Drawing for the job (mm, zero at the part's lowest x, y, z). Give positions to 0.01 mm unless a question says otherwise; leave off trailing zeros. Loops run counter-clockwise (first coordinate to the right, second up) from the corner with the lowest first, then second, coordinate; pieces in that order, holes last.
1) Flat gauge pin, fed straight in: P1, Ø1.4, axis at y = 3, z = 56.857, coming from the +X side. Where does the tip first touch, or does it go through?
2) Band-saw the part on B-B on y = 7. List the corners of the cut face in (x, z), then the cut area to 3 significant figures.
3) Wall check: line 1 (Z direction, x = 0.7, y = 69); line 2 (Y direction, x = 0.95, z = 57); line 3 (Y direction, x = 4.1, z = 15). Give the ranges that are in metal, low to high.
4) Band-saw the part on C-C on x = 4.75. List the corners of the cut face in (y, z), then the cut area to 3 significant figures.
5) Band-saw the part on D-D on z = 32.5. List the corners of the cut face in (x, y).
6) Band-saw the part on A-A on y = 69. List the corners of the cut face in (x, z).
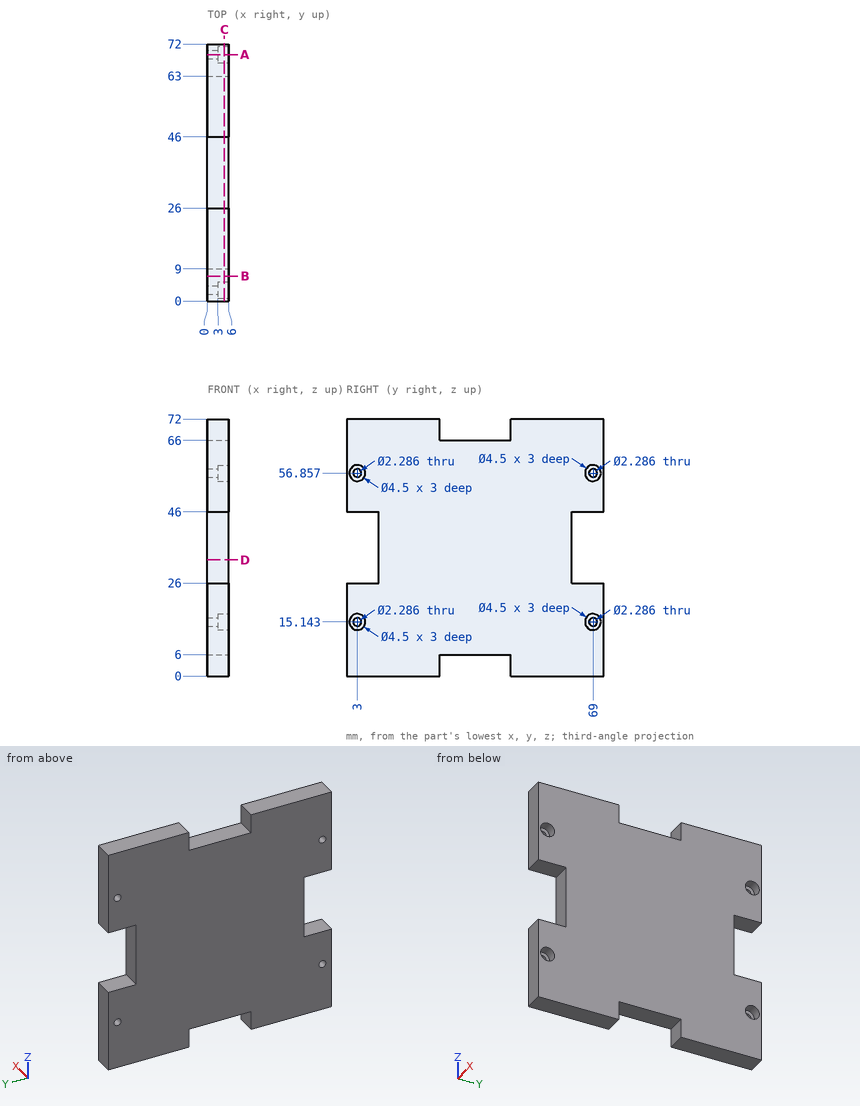
Findings below:
1. P1: passes through
2. outline: (0, 0) - (6, 0) - (6, 26) - (0, 26) - close; (0, 46) - (6, 46) - (6, 72) - (0, 72) - close
2. area: 312 mm2
3. line 1: z = 0 to 14, 16.29 to 26, 46 to 55.71, 58 to 72
3. line 2: y = 0 to 1.87, 4.13 to 67.87, 70.13 to 72
3. line 3: y = 0 to 0.75, 5.25 to 66.75, 71.25 to 72
4. outline: (0, 0) - (26, 0) - (26, 6) - (46, 6) - (46, 0) - (72, 0) - (72, 26) - (63, 26) - (63, 46) - (72, 46) - (72, 72) - (46, 72) - (46, 66) - (26, 66) - (26, 72) - (0, 72) - (0, 46) - (9, 46) - (9, 26) - (0, 26) - close; hole circle Ø4.5 at (3, 15.14); hole circle Ø4.5 at (3, 56.86); hole circle Ø4.5 at (69, 15.14); hole circle Ø4.5 at (69, 56.86)
4. area: 4,520 mm2
5. outline: (0, 9) - (6, 9) - (6, 63) - (0, 63) - close
6. outline: (0, 0) - (6, 0) - (6, 12.89) - (3, 12.89) - (3, 14) - (0, 14) - close; (0, 16.29) - (3, 16.29) - (3, 17.39) - (6, 17.39) - (6, 26) - (0, 26) - close; (0, 46) - (6, 46) - (6, 54.61) - (3, 54.61) - (3, 55.71) - (0, 55.71) - close; (0, 58) - (3, 58) - (3, 59.11) - (6, 59.11) - (6, 72) - (0, 72) - close
